Design review of the part built by this model. Coordinates are the model's own, in mm. Face numbers are marked on the shaded views. A direction names the side the tool comes from. Coordinates: 2 decimals unless noted, no trailing zeros. Loops run counter-clockwise (first coordinate to the right, second up) from the corner with the lowest first, then second, coordinate; pieces in that order, holes last. Notation, with made-up numbers: (59.25, 45) -> (66.25, 45) arc R35 ccw to (66.25, 84) -> close; hole circle Ø7 at (-6.75, 21). An arc over 180 degrees is marked (long way). One line per item, written item: value. Start each with the question number.
1. Add section D-D on z = 14.5. Write out the cut boundary in (x, y).
2. Machinability: for the marked faces 1 and 2, which of the approach directions +Z, -Z, +X, -X, +Y, -Y give a long, thin tool a straight path to every point of the face, cutting with its end or side? Answer none if there is none.
3. For probe 1 along X at (y, z) = (27, 20.5); probe 2 along X at (y, z) = (19, 36); probe 3 along Y at (x, z) = (19, 5.5), list the stretches that pass through material, from the lowest coordinate up.
4. Add section A-A on z = 8.75. Write out the cut boundary in (x, y), plus the area to 3 significant figures.
5. Add section C-C on y = 14.5. Write out the cut boundary in (x, z).
6. Insertion check: pin 1 (5 mm diameter, centred on x = 11, z = 9, fed in from -Y); pin 2 (5 mm diameter, centred on y = 14.5, z = 8.75, fed in from -X). Each pin has a flat end and moves straight along its axis. Give the tip position at first contact, or say it passes through.
7. Add section B-B on y = 7. Write out the cut boundary in (x, z).
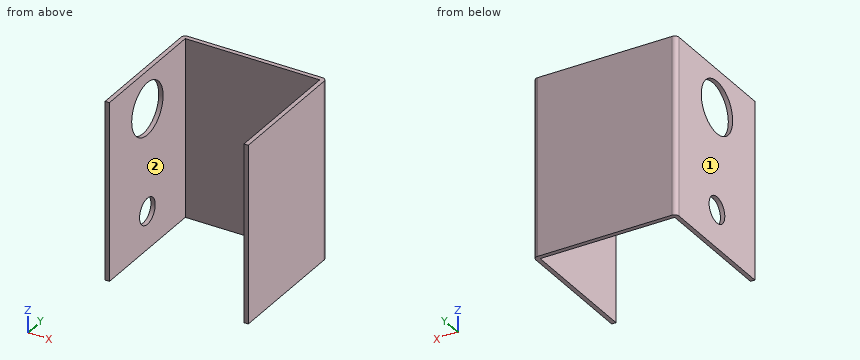
```python
from build123d import *

# Parameters (mm, degrees)
EKSTR_ZYON_NCE1_DEPTH = 41
IZIM2_R               = 3
KES_EKSTR_ZYON1_DEPTH = 5
IZIM4_R               = 6
KES_EKSTR_ZYON3_DEPTH = 22


with BuildPart() as part:
    # Çizim1 → Ekstrüzyon-İnce1 (new body)
    with BuildSketch(Plane.XY):
        with BuildLine():
            Line((0, 0), (0, 29))
            ThreePointArc((0, 29), (0.292893219, 29.707106781), (1, 30))
            Line((1, 30), (32, 30))
            ThreePointArc((32, 30), (32.707106781, 29.707106781), (33, 29))
            Line((33, 29), (33, 0))
            Line((33, 0), (32, 0))
            Line((32, 0), (32, 29))
            Line((32, 29), (1, 29))
            Line((1, 29), (1, 0))
            Line((1, 0), (0, 0))
        make_face()
    extrude(amount=EKSTR_ZYON_NCE1_DEPTH)

    # Çizim2 → Kes-Ekstrüzyon1 (cut)
    with BuildSketch(Plane(origin=(0, 0, 0), x_dir=(0, 0, -1), z_dir=(1, 0, 0))):
        with Locations((-32.25, 14.5)):
            Circle(IZIM2_R)
        with Locations((-8.75, 14.5)):
            Circle(IZIM2_R)
    extrude(amount=KES_EKSTR_ZYON1_DEPTH, mode=Mode.SUBTRACT)

    # Çizim4 → Kes-Ekstrüzyon3 (cut)
    with BuildSketch(Plane.ZY):
        with Locations((32.25, 14.5)):
            Circle(IZIM4_R)
    extrude(amount=-KES_EKSTR_ZYON3_DEPTH, mode=Mode.SUBTRACT)


solid = part.part
```
Worked answers:
1. outline: (0, 0) -> (1, 0) -> (1, 29) -> (32, 29) -> (32, 0) -> (33, 0) -> (33, 29) arc R1 ccw to (32, 30) -> (1, 30) arc R1 ccw to (0, 29) -> close
2. face 1: +Z, -Z, -X, +Y, -Y
2. face 2: +Z, -Z, -Y
3. probe 1: x = 0 to 1, 32 to 33
3. probe 2: x = 32 to 33
3. probe 3: y = 29 to 30
4. outline: (0, 0) -> (1, 0) -> (1, 11.5) -> (0, 11.5) -> close; (0, 17.5) -> (1, 17.5) -> (1, 29) -> (32, 29) -> (32, 0) -> (33, 0) -> (33, 29) arc R1 ccw to (32, 30) -> (1, 30) arc R1 ccw to (0, 29) -> close
4. area: 84.6 mm²
5. outline: (0, 0) -> (1, 0) -> (1, 5.75) -> (0, 5.75) -> close; (0, 11.75) -> (1, 11.75) -> (1, 26.25) -> (0, 26.25) -> close; (0, 38.25) -> (1, 38.25) -> (1, 41) -> (0, 41) -> close; (32, 0) -> (33, 0) -> (33, 41) -> (32, 41) -> close
6. pin 1: stops at y = 29
6. pin 2: stops at x = 32
7. outline: (0, 0) -> (1, 0) -> (1, 41) -> (0, 41) -> close; (32, 0) -> (33, 0) -> (33, 41) -> (32, 41) -> close
